Can you work these out from the drawing? Everything is in mm from the part's minimum corner. Coordinates: 2 decimals unless noted, no trailing zeros. Order: outer loops, then holes, each group sorted by start corner. A loop starts at its lowest first (then second) coordinate and runs counter-clockwise, first axis right, second up. Notation, with made-up numbers: (-29.75, 41.25) -> (-8.75, 41.25) arc R11 ccw to (-8.75, 61.25) -> close; hole circle Ø6 at (-19.75, 89). An arc over 180 degrees is marked (long way). Use a Markdown table: item, result. Add a question column.
1) If I drill on L1, parallel to X at y = 9, z = 3.55; L2, parallel to X at y = 15, z = 3.9; L3, parallel to X at y = 5.25, z = 0.4, over which ranges is the centre line in solid material (lowest first)? Write a range as [from, to].
2) If we section it at A-A (y = 18.5): Write out the boundary of the cut face in (x, z), plus the area to 3 significant figures.
3) Will this pin go through, and if not, where does the flat tip stop? pin 1 Ø3 at (y, z) = (12, 4) entering from -X.
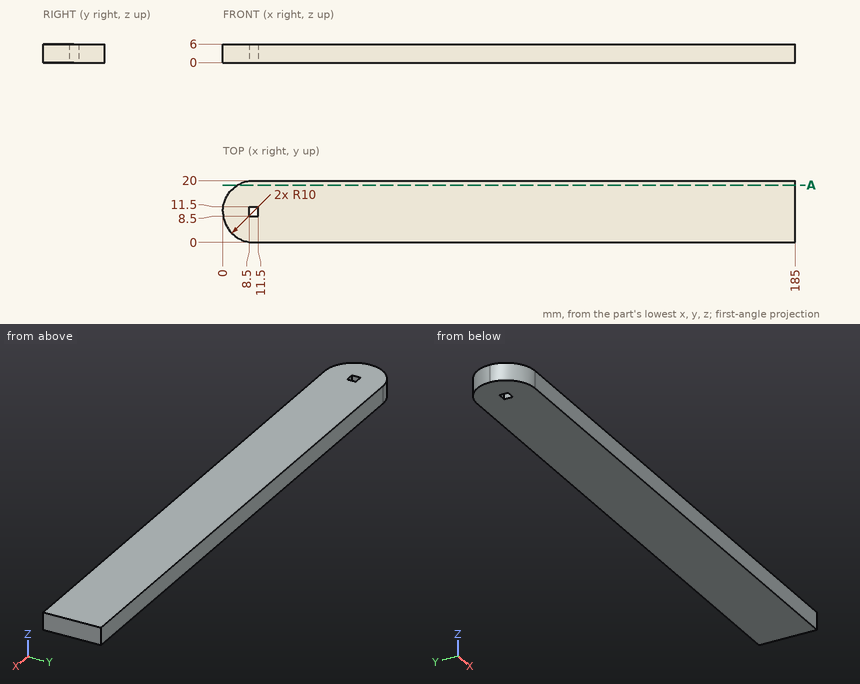
Answer sheet:
| question | item | result |
|---|---|---|
| 1 | L1 | [0.05, 8.5], [11.5, 185] |
| 1 | L2 | [1.34, 185] |
| 1 | L3 | [1.2, 185] |
| 2 | outline | (4.73, 0) -> (185, 0) -> (185, 6) -> (4.73, 6) -> close |
| 2 | area | 1,080 mm2 |
| 3 | pin 1 | x = 0.01 |
